Check sheet for the drawn part. Datum: minimum x, y, z corner. Units: mm. A direction names the side the tool comes from. Give positions to 0.01 mm unless a question says otherwise; leave off trailing zeros. Write each loop counter-clockwise with the first axis right and the second up, starting at its lowest first coordinate (ties: lowest second). Pieces come first, ordered by that corner, then holes. Notation, with made-up numbers: M 0,-20.75 L 21,-20.75 A16 cw 21,-6.75 Z; hole C 78,38.25 d2. An arc over 180 degrees is marked long. Write item = value, one per line. Start each with the question number.
1) Sectioned sample at A-A, the plane x = 3. Record the cut outline in (y, z).
2) Gauge pin test, flat ends, axial feed: pin 1 (1 mm diameter, centred on x = 12.5, y = 7.5, fed in from -Z); pin 2 (3 mm diameter, centred on x = 3, z = 5, fed in from -Y); pin 3 (5 mm diameter, centred on y = 25.5, z = 1.5, fed in from +X); pin 4 (4 mm diameter, centred on y = 10, z = 4, fed in from -X). Record the tip position at first contact, or that the pin passes through.
3) Sectioned sample at C-C, the plane z = 5. Count the separate pieces of the cut face and the enclosed holes in it, then the cut area to 3 significant figures.
4) Sectioned sample at D-D, the plane y = 14. Record the cut outline in (x, z).
5) Draft check along Z on the marked faces 1, 2, 3 and 4. Enter one of: pulls with the +Z half, pulls with the -Z half, needs draft (parallel to the pull), parting line crosses it, or undercut.
6) Sectioned sample at B-B, the plane y = 24. Record the cut outline in (x, z), then the cut area to 3 significant figures.
7) Set-up check for the marked faces 5, 6 and 7: record each of +Z, -Z, +X, -X, +Y, -Y from which the full face is reachable in a straight line by a thin tool's end or side.
8) Scan lines: L1, parallel to X at y = 21, z = 9; L2, parallel to Z at x = 22.5, y = 23; L3, parallel to Y at x = 27, z = 2. Record each from-to range of solid material in increasing order.
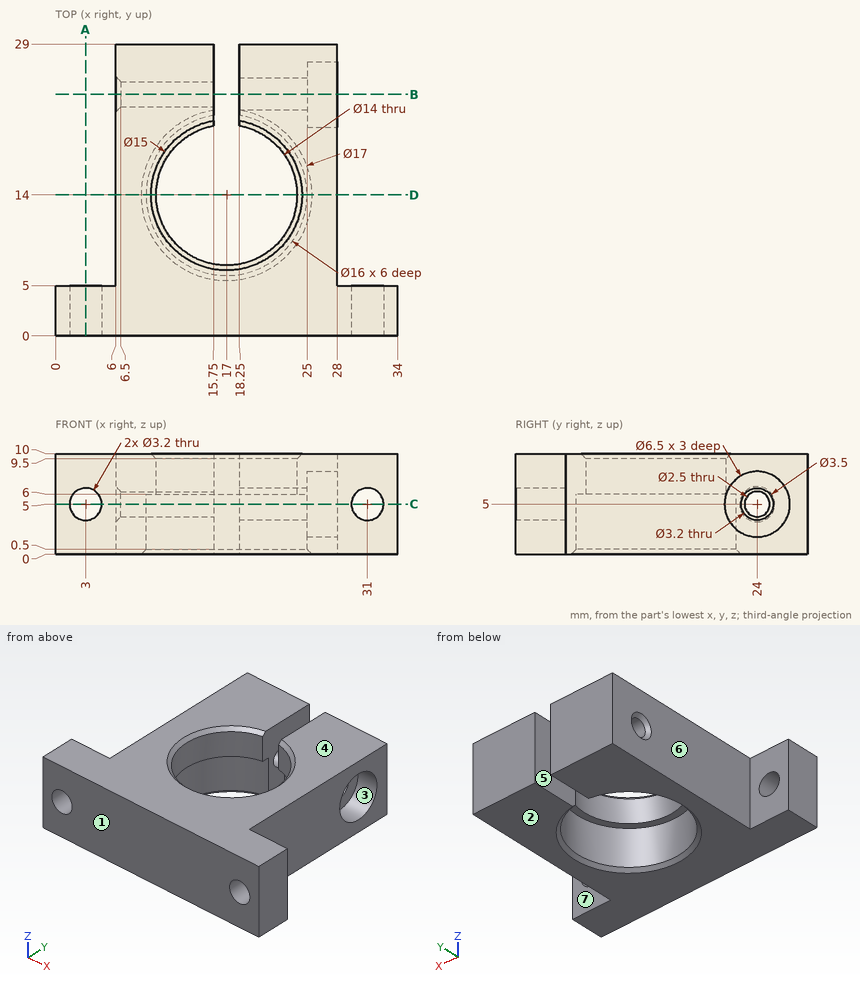
Data:
q1.outline = M 0,0 L 5,0 L 5,3.4 L 0,3.4 Z; M 0,6.6 L 5,6.6 L 5,10 L 0,10 Z
q2.pin_1 = 0.09
q2.pin_2 = through
q2.pin_3 = 28
q2.pin_4 = 6
q3.separate_pieces = 5
q3.enclosed_holes = 0
q3.area = 382 mm2
q4.outline = M 6,0 L 8.5,0 L 9,0.5 L 9,6 L 10,6 L 10,9.5 L 9.5,10 L 6,10 Z; M 24,6 L 25,6 L 25,0.5 L 25.5,0 L 28,0 L 28,10 L 24.5,10 L 24,9.5 Z
q5.face_1 = needs draft
q5.face_2 = pulls with the -Z half
q5.face_3 = undercut
q5.face_4 = pulls with the +Z half
q6.outline = M 6,0 L 15.75,0 L 15.75,3.75 L 6.5,3.75 L 6,3.25 Z; M 6,6.75 L 6.5,6.25 L 15.75,6.25 L 15.75,10 L 6,10 Z; M 18.25,0 L 28,0 L 28,1.75 L 25,1.75 L 25,3.4 L 18.25,3.4 Z; M 18.25,6.6 L 25,6.6 L 25,8.25 L 28,8.25 L 28,10 L 18.25,10 Z
q6.area = 129 mm2
q7.face_5 = +Z, -Z, +Y
q7.face_6 = +Z, -Z, -X, +Y
q7.face_7 = +Z, -Z, +X, +Y
q8.L1 = 6 to 15.75, 18.25 to 28
q8.L2 = 0 to 3.75, 6.25 to 10
q8.L3 = 0 to 22.75, 25.25 to 29
